For this review, use the dimensioned drawing (mm, ordinates from the lowest corner) and the shaded views. A direction names the side the tool comes from. Coordinates: 2 decimals unless noted, no trailing zeros. Write each loop counter-clockwise with the first axis right and the second up, starting at its lowest first coordinate (ties: lowest second). Pieces come first, ordered by that corner, then holes.
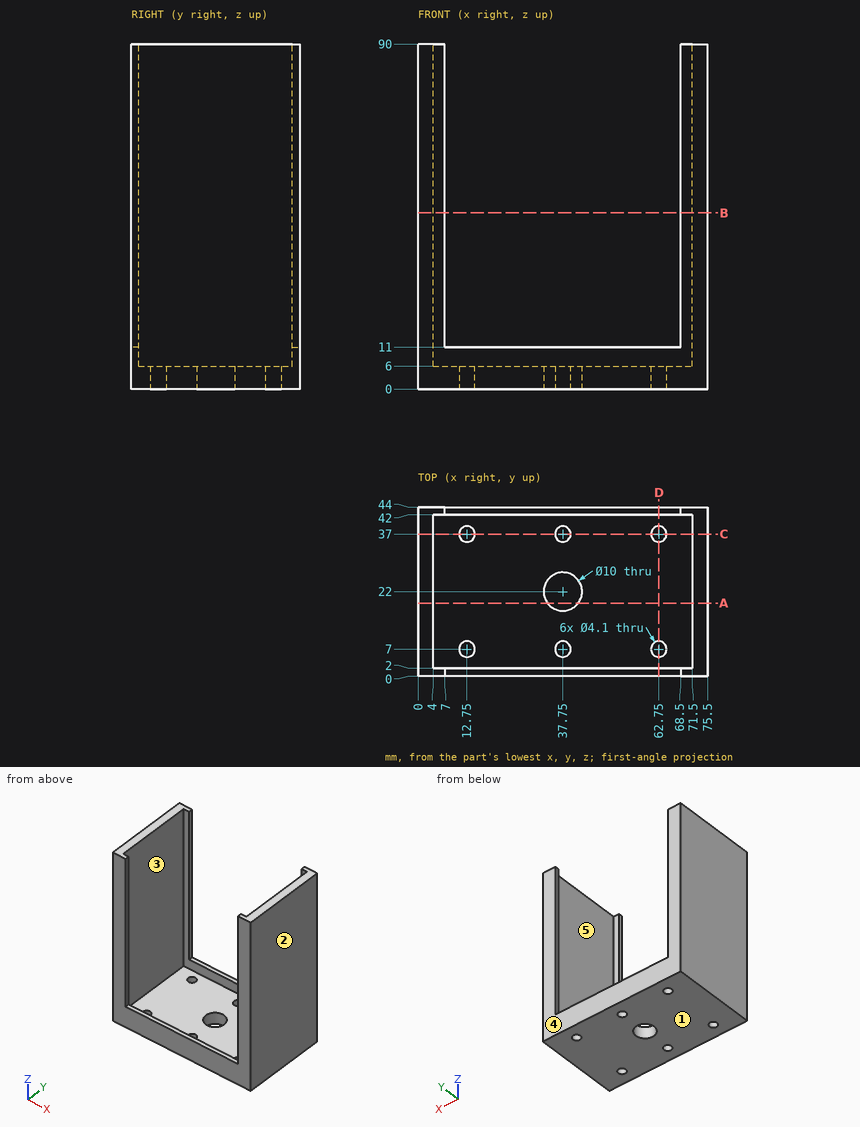
Item 1: Take a section at A-A, the plane y = 19. Write out the cut boundary in (x, z).
Solved:
outline: (0, 0) - (33.75, 0) - (33.75, 6) - (4, 6) - (4, 90) - (0, 90) - close; (41.75, 0) - (75.5, 0) - (75.5, 90) - (71.5, 90) - (71.5, 6) - (41.75, 6) - close
Item 2: Take a section at C-C, the plane y = 37. Write out the cut boundary in (x, z), plus the area to 3 significant figures.
Solved:
outline: (0, 0) - (10.7, 0) - (10.7, 6) - (4, 6) - (4, 90) - (0, 90) - close; (14.8, 0) - (35.7, 0) - (35.7, 6) - (14.8, 6) - close; (39.8, 0) - (60.7, 0) - (60.7, 6) - (39.8, 6) - close; (64.8, 0) - (75.5, 0) - (75.5, 90) - (71.5, 90) - (71.5, 6) - (64.8, 6) - close
area: 1,050 mm2
Item 3: Mouldability with a two-part tool opening along X and no side actions: class the marked faces 1, 2 and 3 as pulls with the +X half, pulls with the -X half, needs draft (parallel to the pull), parting line crosses it, or undercut.
Solved:
face 1: needs draft
face 2: pulls with the +X half
face 3: undercut
Item 4: Take a section at B-B, the plane z = 46. Write out the cut boundary in (x, y), plus the area to 3 significant figures.
Solved:
outline: (0, 0) - (7, 0) - (7, 2) - (4, 2) - (4, 42) - (7, 42) - (7, 44) - (0, 44) - close; (68.5, 0) - (75.5, 0) - (75.5, 44) - (68.5, 44) - (68.5, 42) - (71.5, 42) - (71.5, 2) - (68.5, 2) - close
area: 376 mm2
Item 5: Machinability: for the marked faces 4 and 5, which of the approach directions +Z, -Z, +X, -X, +Y, -Y give a long, thin tool a straight path to every point of the face, cutting with its end or side? Answer none if there is none.
Solved:
face 4: +Z, -Z, +X, -X, +Y
face 5: +Z
Item 6: For pin 1 (12 mm diameter, centred on x = 14.5, y = 35.5, fed in from +Z); pin 2 (0.6 mm diameter, centred on x = 48.5, y = 42.5, fed in from +Z), all flat-tipped, find the tip position at first contact; note any pin that passes through.
Solved:
pin 1: stops at z = 6
pin 2: stops at z = 11
Item 7: To check wall thickness, follow line 1 along Y through (x, z) = (37.75, 2.2); line 2 along Y through (x, z) = (12.75, 3.2); line 3 along X through (y, z) = (32, 76.5). State the ranges of each line that lie inside material, in increasing order.
Solved:
line 1: y = 0 to 4.95, 9.05 to 17, 27 to 34.95, 39.05 to 44
line 2: y = 0 to 4.95, 9.05 to 34.95, 39.05 to 44
line 3: x = 0 to 4, 71.5 to 75.5
Item 8: Take a section at D-D, the plane x = 62.75. Write out the cut boundary in (y, z).
Solved:
outline: (0, 0) - (4.95, 0) - (4.95, 6) - (2, 6) - (2, 11) - (0, 11) - close; (9.05, 0) - (34.95, 0) - (34.95, 6) - (9.05, 6) - close; (39.05, 0) - (44, 0) - (44, 11) - (42, 11) - (42, 6) - (39.05, 6) - close
